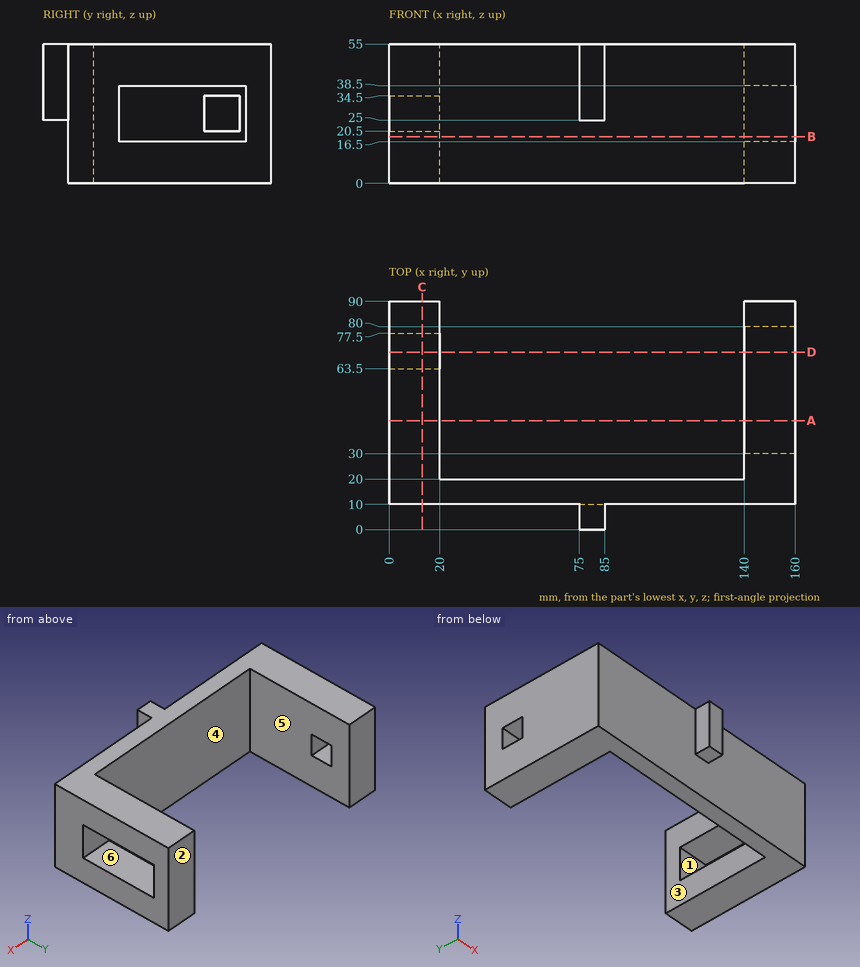
Source: three-view drawing plus pictorial views. Frame: mm from the lowest corner of the part. A direction names the side the tool comes from. Give positions to 0.01 mm unless a question says otherwise; leave off trailing zeros. Order: outer loops, then holes, each group sorted by start corner. A loop starts at its lowest first (then second) coordinate and runs counter-clockwise, first axis right, second up. Notation, with made-up numbers: M 81,14 L 89,14 A22 ccw 89,50 Z; hole C -12,-30 d3. An arc over 180 degrees is marked long. One line per question, with ' | ' between items. Start each with the question number.
1. Section query B-B (z = 18.5). Return the cut outline in (x, y), and give its area (3 significant figures).
2. Material intervals for probe 1 along X at (y, z) = (29.5, 13); probe 2 along Y at (x, z) = (9, 26); probe 3 along Z at (x, y) = (142, 71.5), sorted ascending. Write a range as [from, to].
3. Pull-direction query (Y, two-part tool) for the marked faces 4, 5 and 6; classes: released by +Y, released by -Y, zero draft, split by the parting line, or undercut.
4. Access query for the marked faces 1, 2 and 3. Directions: +Z, -Z, +X, -X, +Y, -Y. A direction counts if a zero-diameter tool reaches every point of the face in a straight line with its end or side. Return the directions, or none.
5. Section query A-A (y = 43). Return the cut outline in (x, z), and give its area (3 significant figures).
6. Section query D-D (y = 70). Return the cut outline in (x, z).
7. Section query C-C (x = 13). Return the cut outline in (y, z).
8. First-contact query: pin 1 Ø16.5 at (x, z) = (114, 29.5) entering from -Y; pin 2 Ø8 at (y, z) = (2.5, 41) entering from -X; pin 3 Ø4 at (x, z) = (25.5, 25) entering from +Y; pin 4 Ø1 at (x, y) = (139, 27.5) entering from -Z. Flat tips, straight axial feed; report the tip coordinate or a pass-through.
Here are the results:
1) outline: M 0,10 L 160,10 L 160,30 L 140,30 L 140,20 L 20,20 L 20,90 L 0,90 Z; M 140,80 L 160,80 L 160,90 L 140,90 Z | area: 3,400 mm²
2) probe 1: [0, 20], [140, 160] | probe 2: [10, 63.5], [77.5, 90] | probe 3: [0, 16.5], [38.5, 55]
3) face 4: released by +Y | face 5: zero draft | face 6: undercut
4) face 1: +X | face 2: +Z, -Z, +X, -X, +Y | face 3: +Z, -Z, +Y
5) outline: M 0,0 L 20,0 L 20,55 L 0,55 Z; M 140,0 L 160,0 L 160,16.5 L 140,16.5 Z; M 140,38.5 L 160,38.5 L 160,55 L 140,55 Z | area: 1,760 mm²
6) outline: M 0,0 L 20,0 L 20,20.5 L 0,20.5 Z; M 0,34.5 L 20,34.5 L 20,55 L 0,55 Z; M 140,0 L 160,0 L 160,16.5 L 140,16.5 Z; M 140,38.5 L 160,38.5 L 160,55 L 140,55 Z
7) outline: M 10,0 L 90,0 L 90,55 L 10,55 Z; hole M 63.5,20.5 L 77.5,20.5 L 77.5,34.5 L 63.5,34.5 Z
8) pin 1: y = 10 | pin 2: x = 75 | pin 3: y = 20 | pin 4: through
